```python
from build123d import *

# Parameters (mm, degrees)
BOSS_EXTRUDE1_DEPTH      = 5
F_9_0_9_DIAMETER_HOLE1_D = 9
M4_TAPPED_HOLE1_D        = 3.3
M4_TAPPED_HOLE1_DEPTH    = 11.5
M4_TAPPED_HOLE1_TIP      = 0.991420021
BOSS_EXTRUDE2_DEPTH      = 10
SKETCH8_R                = 5
CUT_EXTRUDE1_DEPTH       = 10
CHAMFER1_SIZE            = 0.5
CHAMFER1_SIZE2           = 0.181985117


with BuildPart() as part:
    # Sketch1 → Boss-Extrude1 (new, symmetric)
    with BuildSketch(Plane(origin=(0, 0, 0), x_dir=(0, 0, -1), z_dir=(1, 0, 0))):
        with BuildLine():
            Line((-18.315233689, 8.034439304), (-35, -30))
            Line((-35, -30), (-35, -40))
            Line((-35, -40), (35, -40))
            Line((35, -40), (35, -30))
            Line((35, -30), (18.315233689, 8.034439304))
            ThreePointArc((18.315233689, 8.034439304), (0, 20), (-18.315233689, 8.034439304))
        make_face()
    extrude(amount=BOSS_EXTRUDE1_DEPTH, both=True)

    # Ø9.0 (9) Diameter Hole1 (through all)
    with Locations(Plane(origin=(5, 0, 0), x_dir=(0, 0, -1), z_dir=(1, 0, 0))):
        with Locations((0, 0)):
            Hole(F_9_0_9_DIAMETER_HOLE1_D / 2)

    # M4 Tapped Hole1
    with Locations(Plane(origin=(0, -40, 0), x_dir=(-1, 0, 0), z_dir=(0, -1, 0))):
        with Locations((0, -25), (0, -10), (0, 10), (0, 25)):
            Hole(M4_TAPPED_HOLE1_D / 2, depth=M4_TAPPED_HOLE1_DEPTH)
            with Locations((0, 0, -(M4_TAPPED_HOLE1_DEPTH + M4_TAPPED_HOLE1_TIP / 2))):  # 118° drill point
                Cone(0, M4_TAPPED_HOLE1_D / 2, M4_TAPPED_HOLE1_TIP, mode=Mode.SUBTRACT)

    # Sketch7 → Boss-Extrude2 (add)
    with BuildSketch(Plane(origin=(5, 0, 0), x_dir=(0, 0, -1), z_dir=(1, 0, 0))):
        with BuildLine():
            Line((-80.9375, 14.970674459), (-1.25, 19.960899278))
            ThreePointArc((-1.25, 19.960899278), (-11.456862756, 16.393300333), (-18.315233689, 8.034439304))
            Line((-18.315233689, 8.034439304), (-35, -30))
            Line((-35, -30), (-35, -40))
            Line((-35, -40), (-86.858127274, -13.340393184))
            ThreePointArc((-86.858127274, -13.340393184), (-94.682373409, 3.070490366), (-80.9375, 14.970674459))
        make_face()
    extrude(amount=-BOSS_EXTRUDE2_DEPTH)

    # Sketch8 → Cut-Extrude1 (cut)
    with BuildSketch(Plane(origin=(5, 0, 0), x_dir=(0, 0, -1), z_dir=(1, 0, 0))):
        with Locations((-80, 0)):
            Circle(SKETCH8_R)
    extrude(amount=-CUT_EXTRUDE1_DEPTH, mode=Mode.SUBTRACT)

    # Chamfer1
    chamfer1_edges = [part.edges().sort_by_distance(p)[0] for p in [
        (-5, 0, 85),
        (5, 0, 85),
    ]]
    chamfer1_side = [part.faces().sort_by_distance(p)[0] for p in [
        (0, 0, 85),
    ]]
    chamfer(chamfer1_edges, length=CHAMFER1_SIZE, length2=CHAMFER1_SIZE2, reference=chamfer1_side[0])


solid = part.part
```
Can you work these out from the model? Positions are in its coordinate system, mm. A direction names the side the tool comes from. Round coordinates to 2 decimals unless told otherwise and drop trailing zeros. Order: outer loops, then holes, each group sorted by start corner. A loop starts at its lowest first (then second) coordinate and runs counter-clockwise, first axis right, second up. Notation, with made-up numbers: (6, 33) -> (31, 33) arc R20 ccw to (31, 47) -> close; hole circle Ø1 at (55, -6). An arc over 180 degrees is marked (long way). Return JSON: item names as keys, results as strings. Group by question number.
1. If we section it at C-C, the plane y = -20.5: Write out the boundary of the cut face in (x, z), then the cut area to 3 significant figures.
2. I need wall thicknesses on line 1 (X direction, y = -32, z = -10); line 2 (Z direction, x = 0, y = -31.5); line 3 (Z direction, x = 0, y = -35). Which ranges of each line are inside material? Lowest first, please. Write a range as [from, to].
3. If we section it at B-B, the plane y = 0: Write out the boundary of the cut face in (x, z), then the cut area to 3 significant figures.
4. Will these pins go through, and if not, where does the flat tip stop? pin 1 (4 mm diameter, centred on x = 0, z = -10, fed in from +Y); pin 2 (3 mm diameter, centred on x = 0, z = 25, fed in from -Y); pin 3 (2.5 mm diameter, centred on x = 0, z = -25, fed in from -Y).
5. If we section it at D-D, the plane z = -16: Write out the boundary of the cut face in (x, y).
6. Which directions (+Z, -Z, +X, -X, +Y, -Y) give clear straight access to the entire face, cutting with the end or side of a thin tool? Please do faces 1 (the face through (-0.215, -34.17, -26.636)), 2 (the face through (0, -35, -35)).
7. If we section it at A-A, the plane z = 0: Write out the boundary of the cut face in (x, y).
8. We'd pull the mould along Y, two halves only. Please class faces 3 (the face through (-0.07, 4.46, -0.59)), 4 (the face through (-0.4, -34.2, -8.4)), 5 (the face through (0.04, -27.68, 9.72)): released by +Y, released by -Y, zero draft, split by the parting line, or undercut.
Output values:
{
 "1": {"outline": "(-5, -30.83) -> (5, -30.83) -> (5, 72.93) -> (-5, 72.93) -> close", "area": "1,040 mm²"},
 "2": {"line 1": "[-5, -1.65], [1.65, 5]", "line 2": "[-35, -26.65], [-23.35, -11.65], [-8.35, 8.35], [11.65, 23.35], [26.65, 51.53]", "line 3": "[-35, -26.65], [-23.35, -11.65], [-8.35, 8.35], [11.65, 23.35], [26.65, 44.73]"},
 "3": {"outline": "(-5, -21.84) -> (5, -21.84) -> (5, -4.5) -> (-5, -4.5) -> close; (-5, 4.5) -> (5, 4.5) -> (5, 74.82) -> (4.5, 75) -> (-4.5, 75) -> (-5, 74.82) -> close; (-5, 85.18) -> (-4.5, 85) -> (4.5, 85) -> (5, 85.18) -> (5, 95) -> (-5, 95) -> close", "area": "978 mm²"},
 "4": {"pin 1": "y = 18.33", "pin 2": "y = -28.41", "pin 3": "y = -28.26"},
 "5": {"outline": "(-5, -40) -> (5, -40) -> (5, 12) -> (-5, 12) -> close"},
 "6": {"face 1": "-Y", "face 2": "-Z, +X, -X, +Y, -Y"},
 "7": {"outline": "(-5, -40) -> (5, -40) -> (5, -4.5) -> (-5, -4.5) -> close; (-5, 4.5) -> (5, 4.5) -> (5, 20) -> (-5, 20) -> close"},
 "8": {"face 3": "undercut", "face 4": "zero draft", "face 5": "released by -Y"}
}
